The model under review builds one solid part; all positions refer to its coordinate system, in mm. Give positions to 0.01 mm unless a question says otherwise; leave off trailing zeros. Order: outer loops, then holes, each group sorted by start corner. A loop starts at its lowest first (then second) coordinate and runs counter-clockwise, first axis right, second up. Notation, with made-up numbers: (4.5, 55.25) -> (43.5, 55.25) arc R33 cw to (43.5, 88.25) -> close; hole circle Ø10 at (-26, 20.25). An arc over 180 degrees is marked (long way). Answer as a JSON object with one key per item and string values. Group by question number.
from build123d import *

# Parameters (mm, degrees)
BOSS_EXTRUDE1_START = -2
BOSS_EXTRUDE1_DEPTH = 2
FILLET1_R           = 12
FILLET2_R           = 5
FILLET3_R           = 5


with BuildPart() as part:
    # Boss-Extrude1: read off the stored shape, not the designer's step
    # Boss-Extrude1 outline → Boss-Extrude1 (new body)
    with BuildSketch(Plane(origin=(0, 0, 0), x_dir=(1, 0, 0), z_dir=(0, 1, 0)).offset(BOSS_EXTRUDE1_START)):
        Polygon((57, 35.118802154), (57, 72.5), (-57, 72.5), (-57, 35.118802154), (-49, 30.5), (-49, -5.5), (-57, -10.118802154), (-57, -45), (-20.618802154, -45), (-16, -37), (16, -37), (20.618802154, -45), (57, -45), (57, -10.118802154), (49, -5.5), (49, 30.5), align=None)
    extrude(amount=BOSS_EXTRUDE1_DEPTH)

    # Fillet1
    fillet1_edges = [part.edges().sort_by_distance(p)[0] for p in [
        (57, -1, 45),
        (-57, -1, 45),
        (-57, -1, -72.5),
        (57, -1, -72.5),
    ]]
    fillet(fillet1_edges, radius=FILLET1_R)

    # Fillet2
    fillet2_edges = [part.edges().sort_by_distance(p)[0] for p in [
        (57, -1, -35.118802154),
        (57, -1, 10.118802154),
        (20.618802154, -1, 45),
        (-20.618802154, -1, 45),
        (-57, -1, 10.118802154),
        (-57, -1, -35.118802154),
    ]]
    fillet(fillet2_edges, radius=FILLET2_R)

    # Fillet3
    fillet3_edges = [part.edges().sort_by_distance(p)[0] for p in [
        (49, -1, -30.5),
        (49, -1, 5.5),
        (16, -1, 37),
        (-16, -1, 37),
        (-49, -1, 5.5),
        (-49, -1, -30.5),
    ]]
    fillet(fillet3_edges, radius=FILLET3_R)


solid = part.part
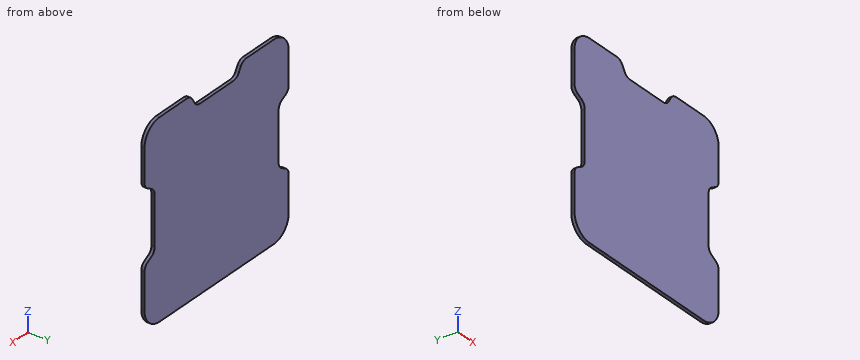
1. For probe 1 along X at (y, z) = (-1.35, -9.5); probe 2 along Z at (x, y) = (52, -0.6); probe 3 along Z at (x, y) = (0.5, -1.4), list the stretches that pass through material, from the lowest coordinate up. Write a range as [from, to].
2. Take a section at B-B on z = -5.5. Give the boundary of the cut face in (x, y), plus the area to 3 significant figures.
3. Take a section at C-C on x = -10. Give the boundary of the cut face in (y, z), plus the area to 3 significant figures.
Checks:
{
 "1": {"probe 1": "x = [-49, 49]", "probe 2": "z = [-70.25, -32.23], [7.23, 42.75]", "probe 3": "z = [-72.5, 37]"},
 "2": {"outline": "(-49, -2) -> (49, -2) -> (49, 0) -> (-49, 0) -> close", "area": "196 mm2"},
 "3": {"outline": "(-2, -72.5) -> (0, -72.5) -> (0, 37) -> (-2, 37) -> close", "area": "219 mm2"}
}
